Verification items for this drawing (mm, ordinates from the low corner). A direction names the side the tool comes from. Round coordinates to 2 decimals unless told otherwise and drop trailing zeros. Loops run counter-clockwise (first coordinate to the right, second up) from the corner with the lowest first, then second, coordinate; pieces in that order, holes last. Notation, with made-up numbers: (-8.75, 44) -> (19.25, 44) arc R33 cw to (19.25, 72) -> close; hole circle Ø5 at (89, 11.5). An arc over 180 degrees is marked (long way). Use a Markdown table: item, result. Add a question column.
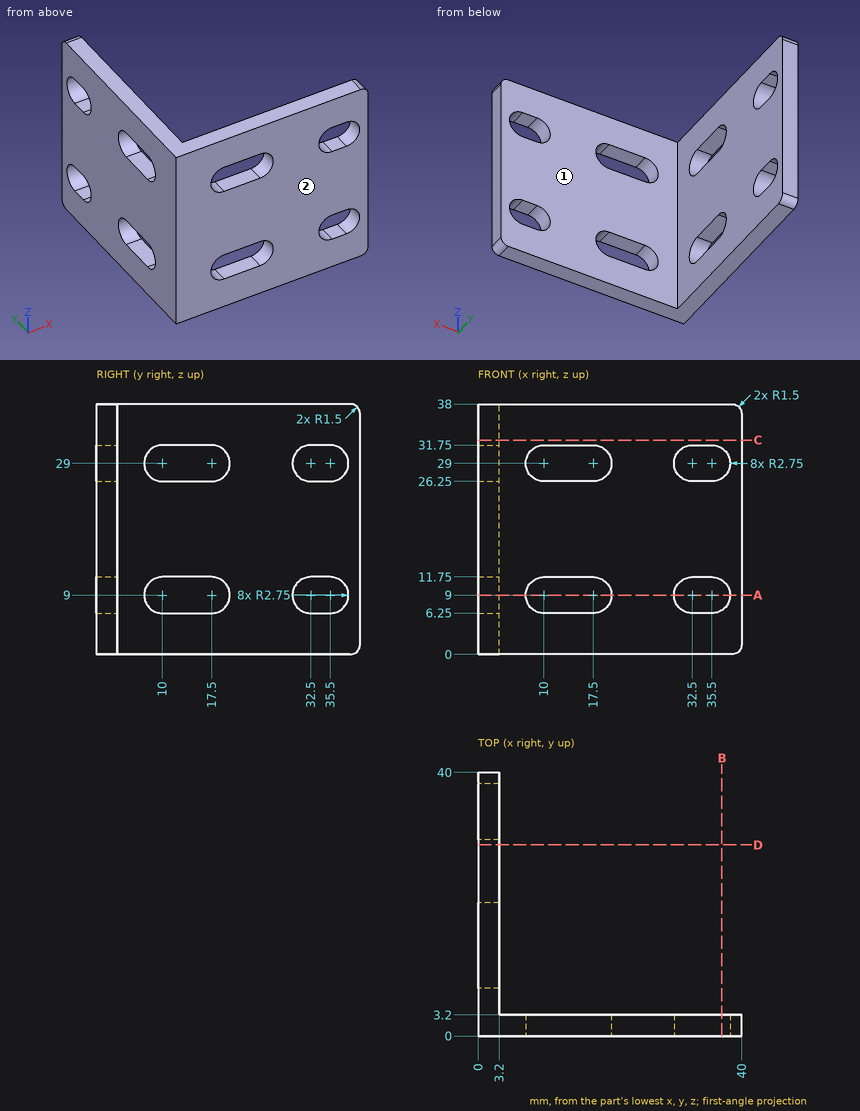
1) Access from +Z, -Z, +X, -X, +Y, -Y to the whole of each face (thin tool, end or side, straight path). Record for the marked faces 1 and 2.
2) Sectioned sample at C-C on z = 32.5. Enter the section's corners in (x, y), then the cut area to 3 significant figures.
3) Sectioned sample at A-A on z = 9. Enter the section's corners in (x, y).
4) Sectioned sample at B-B on x = 37. Enter the section's corners in (y, z).
5) Thickness scan on line 1 (Y direction, x = 3, z = 9); line 2 (X direction, y = 38, z = 27.5). Record the ranges inside material, lowest first.
6) Sectioned sample at D-D on y = 29. Enter the section's corners in (x, z), then the cut area to 3 significant figures.
7) Go/stop test with a flat-tipped pin: pin 1 (2 mm diameter, centred on x = 11, z = 20, fed in from +Y). Record where the tip stops, or that it passes through.
Geometry results:
| question | item | result |
|---|---|---|
| 1 | face 1 | +Z, -Z, +X, +Y |
| 1 | face 2 | +Z, -Z, +X, -X, -Y |
| 2 | outline | (0, 0) -> (40, 0) -> (40, 3.2) -> (3.2, 3.2) -> (3.2, 40) -> (0, 40) -> close |
| 2 | area | 246 mm^2 |
| 3 | outline | (0, 0) -> (7.25, 0) -> (7.25, 3.2) -> (3.2, 3.2) -> (3.2, 7.25) -> (0, 7.25) -> close; (0, 20.25) -> (3.2, 20.25) -> (3.2, 29.75) -> (0, 29.75) -> close; (0, 38.25) -> (3.2, 38.25) -> (3.2, 40) -> (0, 40) -> close; (20.25, 0) -> (29.75, 0) -> (29.75, 3.2) -> (20.25, 3.2) -> close; (38.25, 0) -> (40, 0) -> (40, 3.2) -> (38.25, 3.2) -> close |
| 4 | outline | (0, 0) -> (3.2, 0) -> (3.2, 6.7) -> (0, 6.7) -> close; (0, 11.3) -> (3.2, 11.3) -> (3.2, 26.7) -> (0, 26.7) -> close; (0, 31.3) -> (3.2, 31.3) -> (3.2, 38) -> (0, 38) -> close |
| 5 | line 1 | 0 to 7.25, 20.25 to 29.75, 38.25 to 40 |
| 5 | line 2 | 0 to 3.2 |
| 6 | outline | (0, 0) -> (3.2, 0) -> (3.2, 38) -> (0, 38) -> close |
| 6 | area | 122 mm^2 |
| 7 | pin 1 | y = 3.2 |
